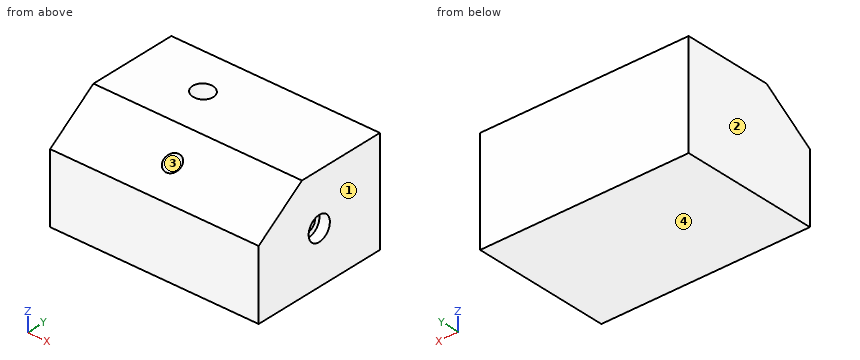
```python
from build123d import *

# Parameters (mm, degrees)
SKETCH_1_W          = 120
SKETCH_1_H          = 80
EXTRUDE_1_DEPTH     = 60
CUT_EXTRUDE_1_DEPTH = 121
SKETCH_5_R          = 7
CUT_EXTRUDE_2_DEPTH = 6
SKETCH_6_R          = 4
CUT_EXTRUDE_3_DEPTH = 50
SWEEP_START         = -57.550317598
SWEEP_6_OUTLINE_R   = 6
SWEEP_6_DEPTH       = 59.776219427
SWEEP_10_PROFILE_R  = 5


# Read off the part's stored shape, not the designer's step: 切除-扫描6
with BuildPart() as part:
    # 草图1 → 凸台-拉伸1 (new body)
    with BuildSketch(Plane.XY):
        with Locations((60, 40)):
            Rectangle(SKETCH_1_W, SKETCH_1_H)
    extrude(amount=EXTRUDE_1_DEPTH)

    # 草图2 → 切除-拉伸1 (cut, symmetric)
    with BuildSketch(Plane(origin=(60, 0, 0), x_dir=(0, 0, -1), z_dir=(1, 0, 0))):
        Polygon((-40, 0), (-60, 0), (-60, 28.5629), align=None)
    extrude(amount=CUT_EXTRUDE_1_DEPTH, both=True, mode=Mode.SUBTRACT)

    # 草图5 → 切除-拉伸2 (cut)
    with BuildSketch(Plane(origin=(120, 0, 0), x_dir=(0, 0, -1), z_dir=(1, 0, 0))):
        with Locations((-30, 40)):
            Circle(SKETCH_5_R)
    extrude(amount=-CUT_EXTRUDE_2_DEPTH, mode=Mode.SUBTRACT)

    # 草图6 → 切除-拉伸3 (cut)
    with BuildSketch(Plane(origin=(120, 0, 0), x_dir=(0, 0, -1), z_dir=(1, 0, 0))):
        with Locations((-30, 40)):
            Circle(SKETCH_6_R)
    extrude(amount=-CUT_EXTRUDE_3_DEPTH, mode=Mode.SUBTRACT)

    # 切除-扫描6 outline → 切除-扫描6 (cut)
    with BuildSketch(Plane(origin=(0, 0, 0), x_dir=(0.9433989278967365, 0.08584365654425449, 0.3203581269054996), z_dir=(0.331660161676509, -0.244180106351077, -0.911250576306588)).offset(SWEEP_START)):
        with Locations((61.67884584, -37.595946176)):
            Circle(SWEEP_6_OUTLINE_R)
    extrude(amount=SWEEP_6_DEPTH, mode=Mode.SUBTRACT)

    # 切除-扫描10: sweep along a curve in space
    with BuildLine() as sweep_10_path:
        Line((57.94, 13.134, 51.638), (57.94, 41.793, 10.709))
    # 切除-扫描10 profile (on start of the path) → 切除-扫描10 (sweep, cut)
    with BuildSketch(Plane(origin=(57.94, 13.134, 51.638), x_dir=(0, -0.8191501102855187, -0.5735791983843407), z_dir=(0, 0.5735791983843407, -0.8191501102855187))):
        Circle(SWEEP_10_PROFILE_R)
    sweep(path=sweep_10_path.line, mode=Mode.SUBTRACT)

    # 草图41 → 切除-放样5 section 0
    with BuildSketch(Plane.XY.offset(8), mode=Mode.PRIVATE) as loft_5_s0:
        with BuildLine():
            Line((64.227, 37.163), (65.185, 39.309))
            Line((65.185, 39.309), (65.19, 41.722))
            Line((65.19, 41.722), (64.24, 44.036))
            Line((64.24, 44.036), (62.483, 45.897))
            Line((62.483, 45.897), (60.183, 47.023))
            Line((60.183, 47.023), (57.692, 47.242))
            Line((57.692, 47.242), (55.389, 46.52))
            Line((55.389, 46.52), (53.625, 44.969))
            Line((53.625, 44.969), (52.667, 42.823))
            Line((52.667, 42.823), (52.662, 40.41))
            Line((52.662, 40.41), (53.612, 38.096))
            Line((53.612, 38.096), (55.37, 36.235))
            Line((55.37, 36.235), (57.669, 35.109))
            Line((57.669, 35.109), (60.16, 34.89))
            Line((60.16, 34.89), (62.463, 35.612))
            Line((62.463, 35.612), (64.227, 37.163))
        make_face()
    loft([loft_5_s0.sketch, Vertex(60.122, 40.186, 4.715)], mode=Mode.SUBTRACT)


solid = part.part
```
For this review, take the finished solid that the model builds, in its own axes (mm). Face numbers are marked on the shaded views. Round coordinates to 2 decimals unless told otherwise and drop trailing zeros. Write each loop counter-clockwise with the first axis right and the second up, starting at its lowest first coordinate (ties: lowest second). Pieces come first, ordered by that corner, then holes. Notation, with made-up numbers: (64, 16.25) - (115, 16.25) arc R12 cw to (115, 20.25) - close; hole circle Ø11 at (68, 77.5). An arc over 180 degrees is marked (long way). Answer as CSV lines item,"result". Start each with the question number.
(1) Add section B-B, the plane z = 30. State how many separate pieces and enclosed holes the cut face has, plus the area to 3 significant figures.
(2) For pin 1 (2 mm diameter, centred on x = 29.5, z = 52, fed in from -Y); pin 2 (12 mm diameter, centred on x = 70.5, z = 51, fed in from -Y); pin 3 (9 mm diameter, centred on y = 40, z = 30, fed in from +X), all flat-tipped, find the tip position at first contact; note any pin that passes through.
(3) Mouldability with a two-part tool opening along X and no side actions: class the marked faces 1, 2, 3 and 4 as +X half, -X half, draft (parallel to the pull), parting line (faces both ways), or undercut.
(4) For line 1 (Y direction, x = 83, z = 30); line 2 (Y direction, x = 116, z = 30); line 3 (Z direction, x = 87.5, y = 39), list the stretches that pass through material, from the lowest coordinate up.
(5) Add section A-A, the plane x = 15. State the section outline as (y, z) points.
From the geometry:
1,separate pieces,"1"
1,enclosed holes,"2"
1,area,"8,940 mm²"
2,pin 1,"stops at y = 15.71"
2,pin 2,"stops at y = 7.14"
2,pin 3,"stops at x = 114"
3,face 1,"+X half"
3,face 2,"-X half"
3,face 3,"undercut"
3,face 4,"draft"
4,line 1,"y = 0 to 36, 44 to 80"
4,line 2,"y = 0 to 33, 47 to 80"
4,line 3,"z = 0 to 26.13, 33.87 to 60"
5,outline,"(0, 0) - (80, 0) - (80, 60) - (28.56, 60) - (0, 40) - close"
